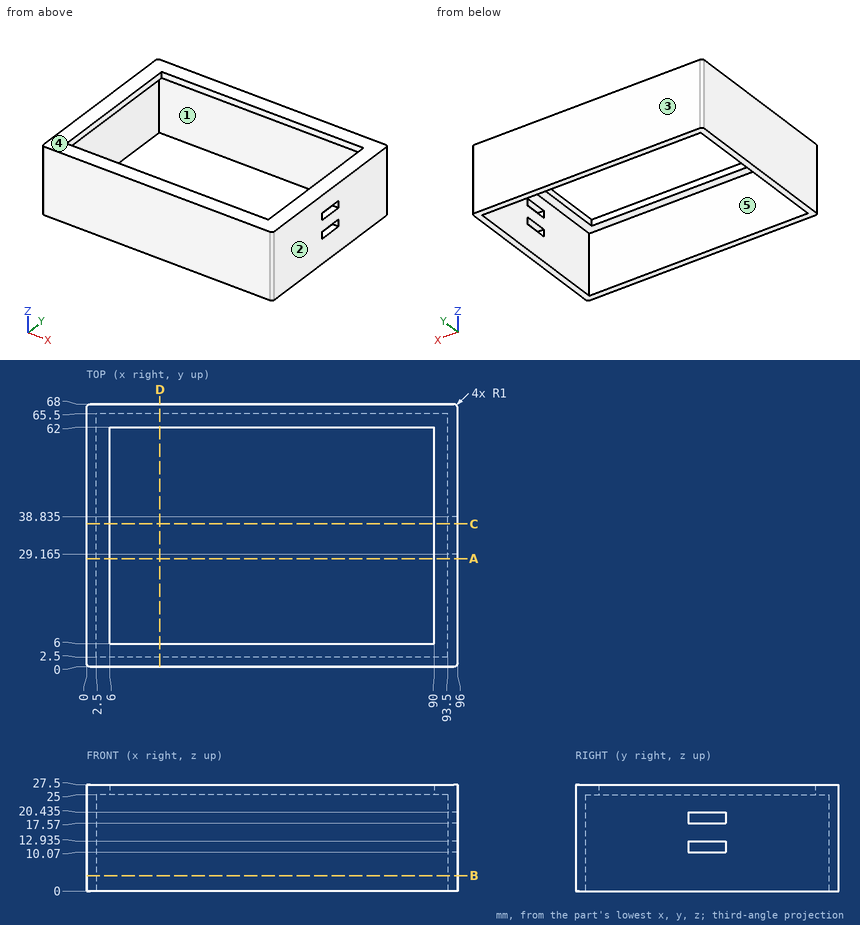
Verification items for this drawing (mm, ordinates from the low corner). A direction names the side the tool comes from. Round coordinates to 2 decimals unless told otherwise and drop trailing zeros. Loops run counter-clockwise (first coordinate to the right, second up) from the corner with the lowest first, then second, coordinate; pieces in that order, holes last. Notation, with made-up numbers: M 40,49.25 L 49,49.25 A18 ccw 49,83.25 Z; hole C 36,86.25 d5. An arc over 180 degrees is marked long. Answer as a JSON object with one key per item and string values.
1. Section check A-A (y = 28). Record the boundary of the cut face in (x, z).
Reply:
{"outline": "M 0,0 L 2.5,0 L 2.5,25 L 6,25 L 6,27.5 L 0,27.5 Z; M 90,25 L 93.5,25 L 93.5,0 L 96,0 L 96,27.5 L 90,27.5 Z"}
2. Mould release check, pull along Y, two halves, no side actions. Record for the marked faces 3, 4 and 5: pulls with the +Y half, pulls with the -Y half, needs draft (parallel to the pull), parting line crosses it, or undercut.
Reply:
{"face 3": "pulls with the +Y half", "face 4": "needs draft", "face 5": "undercut"}
3. Section check C-C (y = 37). Record the boundary of the cut face in (x, z) (1 decimal), plus the area to 3 significant figures.
Reply:
{"outline": "M 0,0 L 2.5,0 L 2.5,25 L 6,25 L 6,27.5 L 0,27.5 Z; M 90,25 L 93.5,25 L 93.5,20.4 L 96,20.4 L 96,27.5 L 90,27.5 Z; M 93.5,0 L 96,0 L 96,10.1 L 93.5,10.1 Z; M 93.5,12.9 L 96,12.9 L 96,17.6 L 93.5,17.6 Z", "area": "141 mm²"}
4. Scan lines: line 1 (Y direction, x = 37.5, z = 21.25); line 2 (X direction, y = 22, z = 3.75); line 3 (Z direction, x = 75, y = 65). Record each from-to range of solid material in increasing order.
Reply:
{"line 1": "y = 0 to 2.5, 65.5 to 68", "line 2": "x = 0 to 2.5, 93.5 to 96", "line 3": "z = 25 to 27.5"}
5. Section check B-B (z = 4). Record the boundary of the cut face in (x, y), plus the area to 3 significant figures.
Reply:
{"outline": "M 0,1 A1 ccw 1,0 L 95,0 A1 ccw 96,1 L 96,67 A1 ccw 95,68 L 1,68 A1 ccw 0,67 Z; hole M 2.5,2.5 L 93.5,2.5 L 93.5,65.5 L 2.5,65.5 Z", "area": "794 mm²"}
6. Section check D-D (x = 19). Record the boundary of the cut face in (y, z), plus the area to 3 significant figures.
Reply:
{"outline": "M 0,0 L 2.5,0 L 2.5,25 L 6,25 L 6,27.5 L 0,27.5 Z; M 62,25 L 65.5,25 L 65.5,0 L 68,0 L 68,27.5 L 62,27.5 Z", "area": "155 mm²"}
7. Access from +Z, -Z, +X, -X, +Y, -Y to the whole of each face (thin tool, end or side, straight path). Record for the marked faces 1 and 2.
Reply:
{"face 1": "-Z", "face 2": "+Z, -Z, +X, +Y, -Y"}
